```python
from build123d import *

# Parameters (mm, degrees)
SKETCH1_R           = 10
BOSS_EXTRUDE1_DEPTH = 41.5
SKETCH2_R           = 2.95
CUT_EXTRUDE1_DEPTH  = 15
SKETCH3_R           = 6
CUT_EXTRUDE2_DEPTH  = 22
CUT_EXTRUDE3_REACH  = 22
SKETCH4_R           = 1.5
SKETCH4_R_2         = 2
CUT_EXTRUDE4_START  = -20
SKETCH4_2_R         = 1.5
SKETCH4_2_R_2       = 2
CUT_EXTRUDE4_DEPTH  = 7.831462


with BuildPart() as part:
    # Sketch1 → Boss-Extrude1 (new body)
    with BuildSketch(Plane.XY):
        Circle(SKETCH1_R)
    extrude(amount=BOSS_EXTRUDE1_DEPTH)

    # Sketch2 → Cut-Extrude1 (cut)
    with BuildSketch(Plane.XY.offset(41.5)):
        Circle(SKETCH2_R)
    extrude(amount=-CUT_EXTRUDE1_DEPTH, mode=Mode.SUBTRACT)

    # Sketch3 → Cut-Extrude2 (cut)
    with BuildSketch(Plane(origin=(0, 0, 0), x_dir=(-1, 0, 0), z_dir=(0, 0, -1))):
        Circle(SKETCH3_R)
    extrude(amount=-CUT_EXTRUDE2_DEPTH, mode=Mode.SUBTRACT)

    # Sketch4 → Cut-Extrude3 (cut, up to next)
    with BuildSketch(Plane.ZY.offset(10), mode=Mode.PRIVATE) as cut_extrude3_sk1:
        with Locations((17, 0)):
            Circle(SKETCH4_R)
    cut_extrude3_tool1 = extrude(cut_extrude3_sk1.sketch, amount=-CUT_EXTRUDE3_REACH, mode=Mode.PRIVATE) & part.part
    add(cut_extrude3_tool1.solids().sort_by_distance((-10, 0, 17))[0], mode=Mode.SUBTRACT)
    # Sketch4 → Cut-Extrude3 (cut, up to next)
    with BuildSketch(Plane.ZY.offset(10), mode=Mode.PRIVATE) as cut_extrude3_sk2:
        with Locations((34, 0)):
            Circle(SKETCH4_R_2)
    cut_extrude3_tool2 = extrude(cut_extrude3_sk2.sketch, amount=-CUT_EXTRUDE3_REACH, mode=Mode.PRIVATE) & part.part
    add(cut_extrude3_tool2.solids().sort_by_distance((-10, 0, 34))[0], mode=Mode.SUBTRACT)

    # Sketch4_2 → Cut-Extrude4 (cut)
    with BuildSketch(Plane.ZY.offset(10).offset(CUT_EXTRUDE4_START)):
        with Locations((17, 0)):
            Circle(SKETCH4_2_R)
        with Locations((34, 0)):
            Circle(SKETCH4_2_R_2)
    extrude(amount=CUT_EXTRUDE4_DEPTH, mode=Mode.SUBTRACT)


solid = part.part
```
Verification items for the finished model (mm, model axes). A direction names the side the tool comes from. Coordinates: 2 decimals unless noted, no trailing zeros. Loops run counter-clockwise (first coordinate to the right, second up) from the corner with the lowest first, then second, coordinate; pieces in that order, holes last. Notation, with made-up numbers: (-0.5, -37) -> (19.5, -37) arc R22 cw to (19.5, -14) -> close; hole circle Ø10 at (-35.5, -12.75). An arc over 180 degrees is marked (long way). Answer in a Markdown table with one row per item.
1) Section check A-A (y = 0). Record the cut outline in (x, z), and give its area (3 significant figures).
The answers:
| item | result |
|---|---|
| outline | (-10, 0) -> (-6, 0) -> (-6, 15.5) -> (-10, 15.5) -> close; (-10, 18.5) -> (-6, 18.5) -> (-6, 22) -> (6, 22) -> (6, 18.5) -> (10, 18.5) -> (10, 32) -> (2.95, 32) -> (2.95, 26.5) -> (-2.95, 26.5) -> (-2.95, 32) -> (-10, 32) -> close; (-10, 36) -> (-2.95, 36) -> (-2.95, 41.5) -> (-10, 41.5) -> close; (2.95, 36) -> (10, 36) -> (10, 41.5) -> (2.95, 41.5) -> close; (6, 0) -> (10, 0) -> (10, 15.5) -> (6, 15.5) -> close |
| area | 397 mm2 |
2) Draft check along Z on faces 1 (the face through (0, -7, 0)), 2 (the face through (-0.64, -2.88, 34.11)), 3 (the face through (-6, 2, 34)). Enter one of: released by +Z, released by -Z, zero draft, split by the parting line, or undercut.
The answers:
| item | result |
|---|---|
| face 1 | released by -Z |
| face 2 | zero draft |
| face 3 | undercut |
3) Scan lines: line 1 along Z through (x, y) = (7.75, 0); line 2 along Y through (x, z) = (0.25, 7); line 3 along X through (y, z) = (0, 31.25). Record each from-to range of solid material in increasing order. Write a range as from..to.
The answers:
| item | result |
|---|---|
| line 1 | z = 0..15.5, 18.5..32, 36..41.5 |
| line 2 | y = -10..-5.99, 5.99..10 |
| line 3 | x = -10..-2.95, 2.95..10 |
4) Section check C-C (x = 8). Record the cut outline in (y, z).
The answers:
| item | result |
|---|---|
| outline | (-6, 0) -> (6, 0) -> (6, 41.5) -> (-6, 41.5) -> close; hole circle Ø4 at (0, 34); hole circle Ø3 at (0, 17) |
5) Access from +Z, -Z, +X, -X, +Y, -Y to the whole of each face (thin tool, end or side, straight path). Record for faces 4 (the face through (0, 0, 26.5)), 5 (the face through (-5.723, 1.802, 10.846)), 6 (the face through (9.54, 3, 20.46)).
The answers:
| item | result |
|---|---|
| face 4 | +Z |
| face 5 | -Z |
| face 6 | +Z, -Z |
6) Depth check by flat-ended pin: P1, Ø5, axis at x = -6, z = 15.5, coming from the -Y side; P2, Ø1.5, axis at x = -5, z = 17, coming from the -Y side; P3, Ø1, axis at x = -3.5, z = 12.5, coming from the +Y side. Enter the tip coordinate at first touch or a pass-through.
The answers:
| item | result |
|---|---|
| P1 | stops at y = -9.37 |
| P2 | stops at y = -9.05 |
| P3 | stops at y = 9.54 |
7) Section check B-B (z = 11.5). Record the cut outline in (x, y).
The answers:
| item | result |
|---|---|
| outline | circle Ø20 at (0, 0); hole circle Ø12 at (0, 0) |
8) Section check D-D (z = 18). Record the cut outline in (x, y), and give its area (3 significant figures).
The answers:
| item | result |
|---|---|
| outline | (-9.94, -1.12) arc R10 ccw to (9.94, -1.12) -> (5.89, -1.12) arc R6 cw to (-5.89, -1.12) -> close; (-9.94, 1.12) -> (-5.89, 1.12) arc R6 cw to (5.89, 1.12) -> (9.94, 1.12) arc R10 ccw to start |
| area | 183 mm2 |
